Drawing for the job (mm, zero at the part's lowest x, y, z). Give positions to 0.01 mm unless a question says otherwise; leave off trailing zeros. Order: outer loops, then holes, each group sorted by start corner. A loop starts at its lowest first (then second) coordinate and runs counter-clockwise, first axis right, second up. Notation, with made-up numbers: M -33.75,52.5 L 18.25,52.5 A15 cw 18.25,76.5 Z; hole C 50,-10 d9. An arc over 180 degrees is marked long. Answer as a JSON object with one key per item and string values.
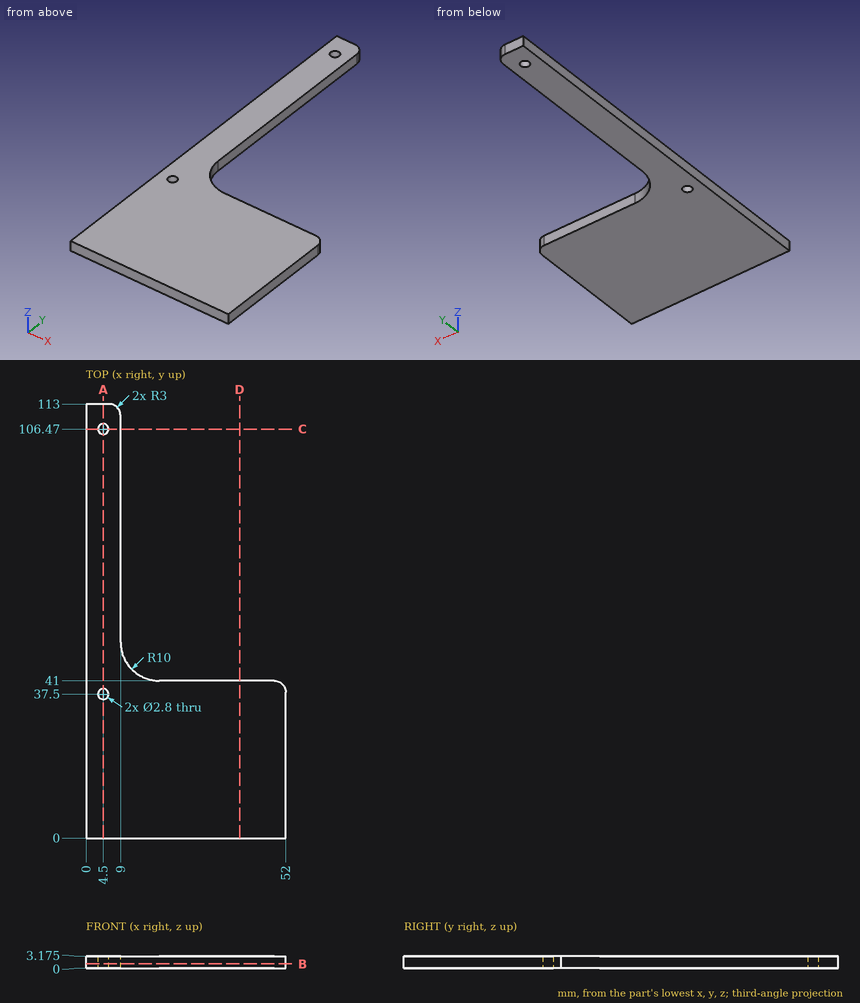
1. Probe line 1 along Y through (x, z) = (4.5, 1.85); line 2 along X through (y, z) = (106.47, 2.45); line 3 along X through (y, z) = (58, 1.5). List the from-to ranges inside material, lowest first.
Worked answers:
{"line 1": "y = 0 to 36.1, 38.9 to 105.07, 107.87 to 113", "line 2": "x = 0 to 3.1, 5.9 to 9", "line 3": "x = 0 to 9"}
2. Pin check, flat tips, straight feed: P1, Ø1, axis at y = 68, z = 1.5, coming from the +X side; P2, Ø1.6, axis at x = 29, z = 1, coming from the +Y side. Stop position of each tip, or through.
Worked answers:
{"P1": "stops at x = 9", "P2": "stops at y = 41"}
3. Cut at A-A on x = 4.5. Give the cut face in (y, z) (3 decimals), plus the area to 3 significant figures.
Worked answers:
{"outline": "M 0,0 L 36.1,0 L 36.1,3.175 L 0,3.175 Z; M 38.9,0 L 105.07,0 L 105.07,3.175 L 38.9,3.175 Z; M 107.87,0 L 113,0 L 113,3.175 L 107.87,3.175 Z", "area": "341 mm^2"}
4. Cut at D-D on x = 40. Give the cut face in (y, z) (3 decimals).
Worked answers:
{"outline": "M 0,0 L 41,0 L 41,3.175 L 0,3.175 Z"}
5. Cut at B-B on z = 1.2. Give the cut face in (x, y), plus the area to 3 significant figures.
Worked answers:
{"outline": "M 0,0 L 52,0 L 52,38 A3 ccw 49,41 L 19,41 A10 cw 9,51 L 9,110 A3 ccw 6,113 L 0,113 Z; hole C 4.5,37.5 d2.8; hole C 4.5,106.47 d2.8", "area": "2,790 mm^2"}
6. Cut at C-C on y = 106.47. Give the cut face in (x, z) (3 decimals), plus the area to 3 significant figures.
Worked answers:
{"outline": "M 0,0 L 3.1,0 L 3.1,3.175 L 0,3.175 Z; M 5.9,0 L 9,0 L 9,3.175 L 5.9,3.175 Z", "area": "19.7 mm^2"}
